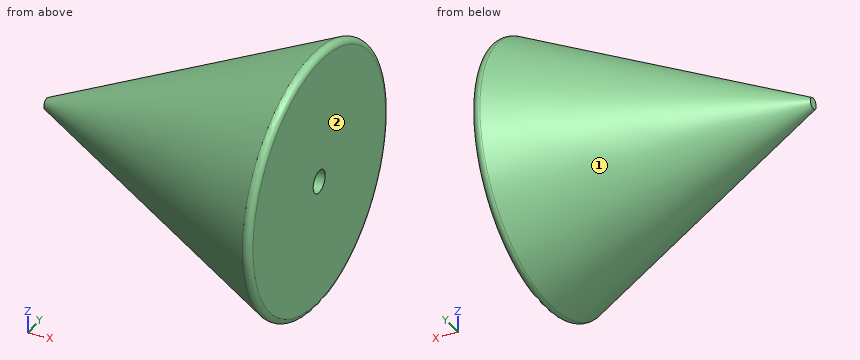
Autodesk Inventor part; units mm, degrees
ref_plane "YZ Plane" through (0, 0, 0) normal (1, 0, 0) x (0, 1, 0)
ref_plane "XZ Plane" through (0, 0, 0) normal (0, 1, 0) x (-1, 0, 0)
ref_plane "XY Plane" through (0, 0, 0) normal (0, 0, 1) x (1, 0, 0)
sketch "Sketch1" plane through (0, 0, 0) normal (0, 0, 1) x (1, 0, 0)
  line L0 (0, 0) -> (0, 26.5512)
  line L1 (0, 26.5512) -> (-55.9167, 26.5512)
  line L2 (-55.9167, 26.5512) -> (0, 0)
  line L3 (-53.8107, 26.5512) -> (-53.8107, 25.5512)
  line L4 (-5, 26.5512) -> (-5, 2.3742)
  dimension "d15" = 1
  dimension "d16" = 5
  dimension "r" = 26.5512
  dimension "d18" = 25.4
  dimension "d19" = 48.8107
revolve "Revolution1" add sketch "Sketch1" angle 360 about axis through (0, 26.5512, 0) along (-1, 0, 0) contours L2 L3 L1 L4
fillet "Fillet1" radius 1 1 edges at (-5, 50.7282, 0)
sketch "Sketch2" plane through (-5, 26.5512, 0) normal (1, 0, 0) x (0, 0, -1)
  circle A0 centre (0, 0) radius 2.05
  circle A1 centre (0, 0) radius 22.5952
  point P0 (0, -26.5512)
  dimension "d7" = 4.1
extrude "Extrusion1" cut sketch "Sketch2" against normal blind 15 contours A0
equation "\"d7\" = dowel + dowelgap"
equation "\"dowel\" = 4"
equation "\"dowelgap\" = 0.1"
properties part number "cone-fixed"
Check sheet for the modelled part. Datum: model origin and axes. Units: mm. Face numbers are marked on the shaded views. Round coordinates to 2 decimals unless told otherwise and drop trailing zeros. Write each loop counter-clockwise with the first axis right and the second up, starting at its lowest first coordinate (ties: lowest second). Pieces come first, ordered by that corner, then holes. Notation, with made-up numbers: M 81.5,68 L 106.5,68 A11 ccw 106.5,79 Z; hole C 61.5,-1.75 d8. An arc over 180 degrees is marked long. Write item = value, one per line. Start each with the question number.
1. Section check D-D, the plane x = -22. Record the cut outline in (y, z), then the cut area to 3 significant figures.
2. Section check C-C, the plane x = -32. Record the cut outline in (y, z).
3. Gauge pin test, flat ends, axial feed: pin 1 (8 mm diameter, centred on x = -46, z = -8, fed in from -Y); pin 2 (12 mm diameter, centred on x = -18, y = 36, fed in from -Z); pin 3 (3 mm diameter, centred on x = -11.5, y = 27, fed in from +Z). Record the tip position at first contact, or that the pin passes through.
4. Scan lines: line 1 (Y direction, x = -8.5, z = -0.5); line 2 (Y direction, x = -13.5, z = 0); line 3 (Z direction, x = -8.5, y = 28). Record each from-to range of solid material in increasing order. Write a range as [from, to].
5. Section check A-A, the plane z = 0. Record the cut outline in (x, y).
6. Release check for a two-part mould opening along X. For the marked faces 1 and 2 record: pulls with the +X half, pulls with the -X half, needs draft (parallel to the pull), parting line crosses it, or undercut.
7. Section check B-B, the plane x = -13.5. Record the cut outline in (y, z).
Results found:
q1.outline = C 26.55,0 d32.21
q1.area = 815 mm^2
q2.outline = C 26.55,0 d22.71
q3.pin_1 = 23.17
q3.pin_2 = -19.43
q3.pin_3 = 21.8
q4.line_1 = [4.04, 24.56], [28.54, 49.06]
q4.line_2 = [6.41, 24.5], [28.6, 46.69]
q4.line_3 = [-22.47, -1.45], [1.45, 22.47]
q5.outline = M -53.81,25.55 L -6.43,3.05 A1 ccw -5,3.96 L -5,24.5 L -20,24.5 L -20,28.6 L -5,28.6 L -5,49.15 A1 ccw -6.43,50.05 L -53.81,27.55 Z
q6.face_1 = pulls with the -X half
q6.face_2 = pulls with the +X half
q7.outline = C 26.55,0 d40.28; hole C 26.55,0 d4.1
